For this review, take the finished solid that the model builds, in its own axes (mm). Face numbers are marked on the shaded views. A direction names the side the tool comes from. Coordinates: 2 decimals unless noted, no trailing zeros. Write each loop counter-clockwise with the first axis right and the second up, starting at its lowest first coordinate (ties: lowest second). Pieces come first, ordered by that corner, then holes. Notation, with made-up numbers: M 56.5,33 L 82.5,33 A11 cw 82.5,47 Z; hole C -37.5,63 d3. An arc over 180 degrees is marked long. One line per question, with ' | ' between items.
from build123d import *

# Parameters (mm, degrees)
BOSS_EXTRUDE1_DEPTH = 25.4
CUT_EXTRUDE1_REACH  = 56.237
SKETCH3_R           = 3.5687
CUT_EXTRUDE2_REACH  = 56.237
SKETCH5_W           = 16.66875
SKETCH5_H           = 42.8625
CUT_EXTRUDE3_DEPTH  = 15.875
BOSS_EXTRUDE2_DEPTH = 4.7625
CUT_EXTRUDE5_REACH  = 65.33
SKETCH9_R           = 1.190625
FILLET1_R           = 0.254
FILLET2_R           = 1.5875


with BuildPart() as part:
    # Sketch2 → Boss-Extrude1 (new body)
    with BuildSketch(Plane.XY):
        Polygon((0, 0), (0, 6.35), (16.66875, 6.35), (16.66875, 36.5125), (0, 36.5125), (0, 42.8625), (21.43125, 42.8625), (21.43125, 0), align=None)
    extrude(amount=BOSS_EXTRUDE1_DEPTH)

    # Sketch3 → Cut-Extrude1 (cut, up to next)
    with BuildSketch(Plane(origin=(21.43125, 0, 0), x_dir=(0, 0, -1), z_dir=(1, 0, 0)), mode=Mode.PRIVATE) as cut_extrude1_sk1:
        with Locations((-19.05, 21.43125)):
            Circle(SKETCH3_R)
    cut_extrude1_tool1 = extrude(cut_extrude1_sk1.sketch, amount=-CUT_EXTRUDE1_REACH, mode=Mode.PRIVATE) & part.part
    add(cut_extrude1_tool1.solids().sort_by_distance((21.43125, 21.43125, 19.05))[0], mode=Mode.SUBTRACT)

    # Sketch4 → Cut-Extrude2 (cut, up to next)
    with BuildSketch(Plane.XY.offset(25.4), mode=Mode.PRIVATE) as cut_extrude2_sk1:
        with BuildLine():
            Line((9.921875, 3.18125), (9.921875, 6.35))
            Line((9.921875, 6.35), (6.746875, 6.35))
            Line((6.746875, 6.35), (6.746875, 3.18125))
            ThreePointArc((6.746875, 3.18125), (8.334375, 1.59375), (9.921875, 3.18125))
        make_face()
    cut_extrude2_tool1 = extrude(cut_extrude2_sk1.sketch, amount=-CUT_EXTRUDE2_REACH, mode=Mode.PRIVATE) & part.part
    # Sketch4 → Cut-Extrude2 (cut, up to next)
    with BuildSketch(Plane.XY.offset(25.4), mode=Mode.PRIVATE) as cut_extrude2_sk2:
        with BuildLine():
            Line((6.746875, 36.5125), (9.921875, 36.5125))
            Line((9.921875, 36.5125), (9.921875, 39.68125))
            ThreePointArc((9.921875, 39.68125), (8.334375, 41.26875), (6.746875, 39.68125))
            Line((6.746875, 39.68125), (6.746875, 36.5125))
        make_face()
    cut_extrude2_tool2 = extrude(cut_extrude2_sk2.sketch, amount=-CUT_EXTRUDE2_REACH, mode=Mode.PRIVATE) & part.part
    add(cut_extrude2_tool1.solids().sort_by_distance((8.334375, 4.127999, 25.4))[0], mode=Mode.SUBTRACT)
    add(cut_extrude2_tool2.solids().sort_by_distance((8.334375, 38.734501, 25.4))[0], mode=Mode.SUBTRACT)

    # Sketch5 → Cut-Extrude3 (cut)
    with BuildSketch(Plane.XY.offset(25.4)):
        with Locations((8.334375, 21.43125)):
            Rectangle(SKETCH5_W, SKETCH5_H)
    extrude(amount=-CUT_EXTRUDE3_DEPTH, mode=Mode.SUBTRACT)

    # Sketch6 → Boss-Extrude2 (add)
    with BuildSketch(Plane(origin=(21.43125, 0, 0), x_dir=(0, 0, -1), z_dir=(1, 0, 0))):
        with BuildLine():
            ThreePointArc((-25.4, 42.8625), (-41.402202947, 21.43125), (-25.4, 0))
            Line((-25.4, 0), (-25.4, 42.8625))
        make_face()
    extrude(amount=-BOSS_EXTRUDE2_DEPTH)

    # Sketch9 → Cut-Extrude5 (cut, up to next)
    with BuildSketch(Plane(origin=(21.43125, 0, 0), x_dir=(0, 0, -1), z_dir=(1, 0, 0)), mode=Mode.PRIVATE) as cut_extrude5_sk1:
        with Locations((-12.05, 21.43125)):
            Circle(SKETCH9_R)
    cut_extrude5_tool1 = extrude(cut_extrude5_sk1.sketch, amount=-CUT_EXTRUDE5_REACH, mode=Mode.PRIVATE) & part.part
    # Sketch9 → Cut-Extrude5 (cut, up to next)
    with BuildSketch(Plane(origin=(21.43125, 0, 0), x_dir=(0, 0, -1), z_dir=(1, 0, 0)), mode=Mode.PRIVATE) as cut_extrude5_sk2:
        with Locations((-19.05, 14.43125)):
            Circle(SKETCH9_R)
    cut_extrude5_tool2 = extrude(cut_extrude5_sk2.sketch, amount=-CUT_EXTRUDE5_REACH, mode=Mode.PRIVATE) & part.part
    # Sketch9 → Cut-Extrude5 (cut, up to next)
    with BuildSketch(Plane(origin=(21.43125, 0, 0), x_dir=(0, 0, -1), z_dir=(1, 0, 0)), mode=Mode.PRIVATE) as cut_extrude5_sk3:
        with Locations((-26.05, 21.43125)):
            Circle(SKETCH9_R)
    cut_extrude5_tool3 = extrude(cut_extrude5_sk3.sketch, amount=-CUT_EXTRUDE5_REACH, mode=Mode.PRIVATE) & part.part
    # Sketch9 → Cut-Extrude5 (cut, up to next)
    with BuildSketch(Plane(origin=(21.43125, 0, 0), x_dir=(0, 0, -1), z_dir=(1, 0, 0)), mode=Mode.PRIVATE) as cut_extrude5_sk4:
        with Locations((-19.05, 28.43125)):
            Circle(SKETCH9_R)
    cut_extrude5_tool4 = extrude(cut_extrude5_sk4.sketch, amount=-CUT_EXTRUDE5_REACH, mode=Mode.PRIVATE) & part.part
    add(cut_extrude5_tool1.solids().sort_by_distance((21.43125, 21.43125, 12.05))[0], mode=Mode.SUBTRACT)
    add(cut_extrude5_tool2.solids().sort_by_distance((21.43125, 14.43125, 19.05))[0], mode=Mode.SUBTRACT)
    add(cut_extrude5_tool3.solids().sort_by_distance((21.43125, 21.43125, 26.05))[0], mode=Mode.SUBTRACT)
    add(cut_extrude5_tool4.solids().sort_by_distance((21.43125, 28.43125, 19.05))[0], mode=Mode.SUBTRACT)

    # Fillet1
    fillet1_edges = [part.edges().sort_by_distance(p)[0] for p in [
        (21.43125, 21.43125, 41.402202947),
        (16.66875, 21.43125, 41.402202947),
        (21.43125, 42.8625, 12.7),
        (21.43125, 0, 12.7),
        (16.66875, 42.8625, 17.4625),
        (16.66875, 0, 17.4625),
    ]]
    fillet(fillet1_edges, radius=FILLET1_R)

    # Fillet2
    fillet2_edges = [part.edges().sort_by_distance(p)[0] for p in [
        (16.66875, 6.35, 4.7625),
        (16.66875, 36.5125, 4.7625),
    ]]
    fillet(fillet2_edges, radius=FILLET2_R)


solid = part.part
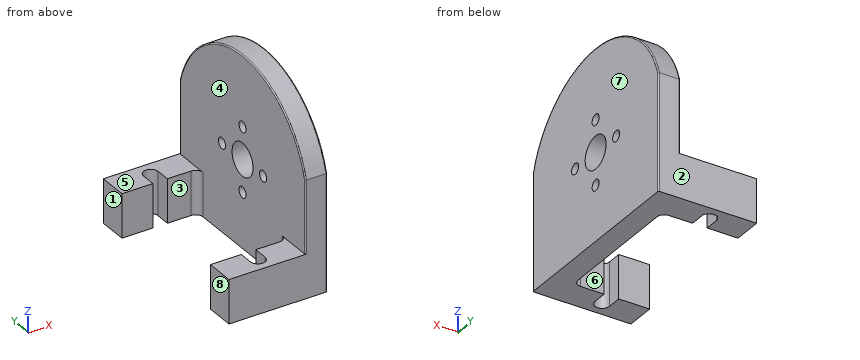
1. Take a section at B-B on z = 12.05. State the section outline as (x, y) points.
Computed values:
outline: M 16.67,0.25 A0.25 ccw 16.92,0 L 21.18,0 A0.25 ccw 21.43,0.25 L 21.43,20.24 L 16.67,20.24 Z; M 16.67,22.62 L 21.43,22.62 L 21.43,42.61 A0.25 ccw 21.18,42.86 L 16.92,42.86 A0.25 ccw 16.67,42.61 Z
2. For line 1 along Y through (x, z) = (20.3, 19.05); line 2 along Y through (x, z) = (1.5, 5); line 3 along X through (y, z) = (2.5, 14.5), list the stretches that pass through material, from the lowest coordinate up.
Computed values:
line 1: y = 0 to 13.24, 15.62 to 17.86, 25 to 27.24, 29.62 to 42.86 | line 2: y = 0 to 6.35, 36.51 to 42.86 | line 3: x = 16.67 to 21.43
3. Draft analysis for pull direction Y (two halves, no side actions). For the marked faces 1, 2 and 3, state which applies: pulls with the +Y half, pulls with the -Y half, needs draft (parallel to the pull), parting line crosses it, or undercut.
Computed values:
face 1: needs draft | face 2: pulls with the +Y half | face 3: undercut
4. Machinability: for the marked faces 4, 5, 6, 7 and 8, which of the approach directions +Z, -Z, +X, -X, +Y, -Y give a long, thin tool a straight path to every point of the face, cutting with its end or side? Answer none if there is none.
Computed values:
face 4: +Z, -X | face 5: +Z, -X, +Y, -Y | face 6: +Z, -Z, -X | face 7: +Z, -Z, +X, +Y, -Y | face 8: +Z, -Z, -X, +Y, -Y
5. Take a section at A-A on z = 19.05. State the section outline as (x, y) points.
Computed values:
outline: M 16.67,0.25 A0.25 ccw 16.92,0 L 21.18,0 A0.25 ccw 21.43,0.25 L 21.43,13.24 L 16.67,13.24 Z; M 16.67,15.62 L 21.43,15.62 L 21.43,17.86 L 16.67,17.86 Z; M 16.67,25 L 21.43,25 L 21.43,27.24 L 16.67,27.24 Z; M 16.67,29.62 L 21.43,29.62 L 21.43,42.61 A0.25 ccw 21.18,42.86 L 16.92,42.86 A0.25 ccw 16.67,42.61 Z
6. Clearance check with flat-ended pins moving along their axes: P1, Ø5.5, axis at x = 3.5, z = 6.5, coming from the -Y side; P2, Ø12, axis at y = 6.5, z = 27.5, coming from the -X side; P3, Ø2.5, axis at x = 10.5, y = 4.5, coming from the +Z side (3 decimals). State where each tip first meets the part, or that it passes through.
Computed values:
P1: stops at y = 0 | P2: stops at x = 16.67 | P3: stops at z = 9.525
